```python
from build123d import *

# Parameters (mm, degrees)
SKETCH1_W                  = 40
SKETCH1_H                  = 22
BOSS_EXTRUDE1_DEPTH        = 11
SKETCH2_W                  = 40
SKETCH2_H                  = 22
SKETCH2_R                  = 7.843750423
BOSS_EXTRUDE2_DEPTH        = 5
SKETCH3_W                  = 24.5
SKETCH3_H                  = 15.5
CUT_EXTRUDE1_DEPTH         = 7.75
FILLET1_R                  = 7.75
SKETCH4_R                  = 5
CUT_EXTRUDE2_DEPTH         = 36.805900352
SKETCH5_W                  = 8
SKETCH5_H                  = 8
SKETCH5_R                  = 1.905800151
BOSS_EXTRUDE3_DEPTH        = 6
CUT_EXTRUDE3_START         = -3
SKETCH6_R                  = 3
SKETCH6_R_2                = 1.905800151
CUT_EXTRUDE3_DEPTH         = 3
SKETCH7_W                  = 16
SKETCH7_H                  = 16.5
BOSS_EXTRUDE5_DEPTH        = 28
MIRROR14_COPY_1_SKETCH_W   = 8
MIRROR14_COPY_1_SKETCH_H   = 8
MIRROR14_COPY_1_SKETCH_R   = 1.905800151
MIRROR14_COPY_1_DEPTH      = 6
MIRROR14_START             = -3
MIRROR14_COPY_2_SKETCH_R   = 3
MIRROR14_COPY_2_SKETCH_R_2 = 1.905800151
MIRROR14_COPY_2_DEPTH      = 3
FILLET1_OF_MIRROR14_R      = 7.75
SKETCH9_W                  = 28
SKETCH9_H                  = 3
BOSS_EXTRUDE6_DEPTH        = 18
CUT_EXTRUDE4_DEPTH         = 10
CUT_EXTRUDE5_DEPTH         = 73.919476136
CUT_EXTRUDE5_DEPTH_BACK    = 73.919476136
SKETCH11_R                 = 1.75
CUT_EXTRUDE6_DEPTH         = 76.121568141
CUT_EXTRUDE6_DEPTH_BACK    = 76.121568141
SKETCH12_R                 = 1.75
CUT_EXTRUDE9_DEPTH         = 12
CUT_EXTRUDE11_START        = -10
SKETCH16_R                 = 4
SKETCH16_R_2               = 1.75
SKETCH16_W                 = 10
SKETCH16_H                 = 6.5
CUT_EXTRUDE11_DEPTH        = 10
FILLET2_R                  = 2


# Some blends are built 0.0001 mm under size
with BuildPart() as part:
    # Sketch1 → Boss-Extrude1 (new body)
    with BuildSketch(Plane(origin=(0, 0, 0), x_dir=(1, 0, 0), z_dir=(0, 1, 0))):
        Rectangle(SKETCH1_W, SKETCH1_H)
    boss_extrude1 = extrude(amount=BOSS_EXTRUDE1_DEPTH)

    # Sketch2 → Boss-Extrude2 (add)
    with BuildSketch(Plane(origin=(0, 0, 0), x_dir=(1, 0, 0), z_dir=(0, 1, 0))):
        Rectangle(SKETCH2_W, SKETCH2_H)
        with Locations(Location((0, 0, 0), (0, 0, 270))):
            Circle(SKETCH2_R, mode=Mode.SUBTRACT)
    boss_extrude2 = extrude(amount=-BOSS_EXTRUDE2_DEPTH)

    # Sketch3 → Cut-Extrude1 (cut)
    with BuildSketch(Plane(origin=(0, 11, 0), x_dir=(1, 0, 0), z_dir=(0, 1, 0))):
        Rectangle(SKETCH3_W, SKETCH3_H)
    cut_extrude1 = extrude(amount=-CUT_EXTRUDE1_DEPTH, mode=Mode.SUBTRACT)

    # Fillet1
    fillet1_edges = [part.edges().sort_by_distance(p)[0] for p in [
        (0, 3.25, 7.75),
        (0, 3.25, -7.75),
    ]]
    fillet(fillet1_edges, radius=FILLET1_R - 0.0001)  # a hair under: the kernel refuses the full size

    # Sketch4 → Cut-Extrude2 (cut, symmetric)
    with BuildSketch(Plane(origin=(-12.25, 0, 0), x_dir=(0, 0, -1), z_dir=(1, 0, 0))):
        with Locations((0, 11)):
            Circle(SKETCH4_R)
    cut_extrude2 = extrude(amount=CUT_EXTRUDE2_DEPTH, both=True, mode=Mode.SUBTRACT)

    # Sketch5 → Boss-Extrude3 (add)
    with BuildSketch(Plane(origin=(0, 11, 0), x_dir=(1, 0, 0), z_dir=(0, 1, 0))):
        with Locations((16, -15)):
            Rectangle(SKETCH5_W, SKETCH5_H)
        with Locations(Location((16, -15, 0), (0, 0, 270))):
            Circle(SKETCH5_R, mode=Mode.SUBTRACT)
    boss_extrude3 = extrude(amount=-BOSS_EXTRUDE3_DEPTH)

    # Sketch6 → Cut-Extrude3 (cut)
    with BuildSketch(Plane.XZ.offset(-5).offset(CUT_EXTRUDE3_START)):
        with Locations(Location((16, 15, 0), (0, 0, 270))):
            Circle(SKETCH6_R)
        with Locations(Location((16, 15, 0), (0, 0, 90))):
            Circle(SKETCH6_R_2, mode=Mode.SUBTRACT)
    cut_extrude3 = extrude(amount=CUT_EXTRUDE3_DEPTH, mode=Mode.SUBTRACT)

    # Mirror8: Boss-Extrude3, Cut-Extrude3 across plane
    add(boss_extrude3.mirror(Plane(origin=(0, 0, 0), x_dir=(0, 0, 1), z_dir=(1, 0, 0))))
    add(cut_extrude3.mirror(Plane(origin=(0, 0, 0), x_dir=(0, 0, 1), z_dir=(1, 0, 0))), mode=Mode.SUBTRACT)

    # Sketch7 → Boss-Extrude5 (add)
    with BuildSketch(Plane(origin=(0, 0, -11), x_dir=(-1, 0, 0), z_dir=(0, 0, -1))):
        with Locations((-12, 9.25)):
            Rectangle(SKETCH7_W, SKETCH7_H)
    extrude(amount=BOSS_EXTRUDE5_DEPTH)

    # Mirror14: Boss-Extrude1, Boss-Extrude2, Cut-Extrude1, Cut-Extrude2, Boss-Extrude3, Cut-Extrude3 across plane
    add(boss_extrude1.mirror(Plane.XY.offset(-25)))
    add(boss_extrude2.mirror(Plane.XY.offset(-25)))
    add(cut_extrude1.mirror(Plane.XY.offset(-25)), mode=Mode.SUBTRACT)
    add(cut_extrude2.mirror(Plane.XY.offset(-25)), mode=Mode.SUBTRACT)
    add(boss_extrude3.mirror(Plane.XY.offset(-25)))
    add(cut_extrude3.mirror(Plane.XY.offset(-25)), mode=Mode.SUBTRACT)

    # Mirror14 copy 1 sketch → Mirror14 copy 1 (add)
    with BuildSketch(Plane(origin=(0, 11, -50), x_dir=(-1, 0, 0), z_dir=(0, 1, 0))):
        with Locations((16, -15)):
            Rectangle(MIRROR14_COPY_1_SKETCH_W, MIRROR14_COPY_1_SKETCH_H)
        with Locations(Location((16, -15, 0), (0, 0, 270))):
            Circle(MIRROR14_COPY_1_SKETCH_R, mode=Mode.SUBTRACT)
    extrude(amount=-MIRROR14_COPY_1_DEPTH)

    # Mirror14 copy 2 sketch → Mirror14 copy 2 (cut)
    with BuildSketch(Plane(origin=(0, 5, -50), x_dir=(-1, 0, 0), z_dir=(0, -1, 0)).offset(MIRROR14_START)):
        with Locations(Location((16, 15, 0), (0, 0, 270))):
            Circle(MIRROR14_COPY_2_SKETCH_R)
        with Locations(Location((16, 15, 0), (0, 0, 90))):
            Circle(MIRROR14_COPY_2_SKETCH_R_2, mode=Mode.SUBTRACT)
    extrude(amount=MIRROR14_COPY_2_DEPTH, mode=Mode.SUBTRACT)

    # Fillet1 of Mirror14
    fillet1_of_mirror14_edges = [part.edges().sort_by_distance(p)[0] for p in [
        (0, 3.25, -57.75),
        (0, 3.25, -42.25),
    ]]
    fillet(fillet1_of_mirror14_edges, radius=FILLET1_OF_MIRROR14_R - 0.0001)  # a hair under: the kernel refuses the full size

    # Sketch9 → Boss-Extrude6 (add)
    with BuildSketch(Plane.ZY.offset(-4)):
        with Locations((-25, 2.5)):
            Rectangle(SKETCH9_W, SKETCH9_H)
    extrude(amount=BOSS_EXTRUDE6_DEPTH)

    # Sketch10 → Cut-Extrude4 (cut)
    with BuildSketch(Plane(origin=(0, 17.5, 0), x_dir=(1, 0, 0), z_dir=(0, 1, 0))):
        with BuildLine():
            Line((9, 26.25), (9, 23.75))
            Line((9, 23.75), (11.727178029, 23.75))
            ThreePointArc((11.727178029, 23.75), (11.931001031, 24.360286817), (12, 25))
            ThreePointArc((12, 25), (11.931001031, 25.639713183), (11.727178029, 26.25))
            Line((11.727178029, 26.25), (9, 26.25))
        make_face()
        with BuildLine():
            Line((11.727178029, 23.75), (9, 23.75))
            Line((9, 23.75), (9, 26.25))
            Line((9, 26.25), (11.727178029, 26.25))
            ThreePointArc((11.727178029, 26.25), (6, 25), (11.727178029, 23.75))
        make_face()
        with BuildLine():
            ThreePointArc((12, 25), (11.931001031, 24.360286817), (11.727178029, 23.75))
            Line((11.727178029, 23.75), (20, 23.75))
            Line((20, 23.75), (20, 26.25))
            Line((20, 26.25), (11.727178029, 26.25))
            ThreePointArc((11.727178029, 26.25), (11.931001031, 25.639713183), (12, 25))
        make_face()
    extrude(amount=-CUT_EXTRUDE4_DEPTH, mode=Mode.SUBTRACT)

    # Sketch11 → Cut-Extrude5 (cut, two sides: drawn at the far end of the back side and taken through both)
    with BuildSketch(Plane(origin=(0, 7.5, 0), x_dir=(1, 0, 0), z_dir=(0, 1, 0)).offset(-CUT_EXTRUDE5_DEPTH_BACK)):
        with Locations(Location((9, 25, 0), (0, 0, 270))):
            Circle(SKETCH11_R)
    extrude(amount=CUT_EXTRUDE5_DEPTH + CUT_EXTRUDE5_DEPTH_BACK, mode=Mode.SUBTRACT)

    # Sketch12 → Cut-Extrude6 (cut, two sides: drawn at the far end of the back side and taken through both)
    with BuildSketch(Plane.ZY.offset(-4).offset(-CUT_EXTRUDE6_DEPTH_BACK)):
        with Locations((-33, 11)):
            Circle(SKETCH12_R)
    extrude(amount=CUT_EXTRUDE6_DEPTH + CUT_EXTRUDE6_DEPTH_BACK, mode=Mode.SUBTRACT)

    # Sketch15 → Cut-Extrude9 (cut)
    with BuildSketch(Plane(origin=(20, 0, 0), x_dir=(0, 0, -1), z_dir=(1, 0, 0))):
        Polygon((33, 14.175426481), (30.25, 12.58771324), (30.25, 9.41228676), (33, 7.824573519), (35.75, 9.41228676), (35.75, 12.58771324), align=None)
    extrude(amount=-CUT_EXTRUDE9_DEPTH, mode=Mode.SUBTRACT)

    # Sketch16 → Cut-Extrude11 (cut)
    # profile 1 of 2: a face of its own
    with BuildSketch(Plane(origin=(20, 0, 0), x_dir=(0, 0, -1), z_dir=(1, 0, 0)).offset(CUT_EXTRUDE11_START)):
        with Locations((33, 11)):
            Circle(SKETCH16_R)
        with Locations((33, 11)):
            Circle(SKETCH16_R_2, mode=Mode.SUBTRACT)
    # profile 2 of 2: a face of its own
    with BuildSketch(Plane(origin=(20, 0, 0), x_dir=(0, 0, -1), z_dir=(1, 0, 0)).offset(CUT_EXTRUDE11_START)):
        with Locations((34, 14.25)):
            Rectangle(SKETCH16_W, SKETCH16_H)
    extrude(amount=CUT_EXTRUDE11_DEPTH, mode=Mode.SUBTRACT)

    # Chamfer3
    # the kernel refuses this chamfer: 2.5 mm, written as the material it takes off along each edge
    with BuildSketch(Plane(origin=(4.790141486, 11, -37), x_dir=(0, -0.9712202897009368, 0.23818301550116588), z_dir=(1, 0, 0))) as chamfer3_piece_1_section:
        with BuildLine():
            Line((1.641163776, 0), (-0.550057664, 2.010038976))
            Line((-0.550057664, 2.010038976), (-0.598618679, 1.998129825))
            ThreePointArc((-0.598618679, 1.998129825), (-0.296653042, 0.999716345), (-0.048561014, -0.011909151))
            Line((-0.048561014, -0.011909151), (0.011909151, -0.048561014))
            ThreePointArc((0.011909151, -0.048561014), (0.818444442, 0.062835502), (1.633479525, -0.049405994))
            Line((1.633479525, -0.049405994), (1.641163776, 0))
        make_face()
    chamfer3_piece_1 = extrude(amount=20.419717028, mode=Mode.PRIVATE)
    chamfer3_piece_1 = split(chamfer3_piece_1, bisect_by=Plane(origin=(10, 11.063270064, -39.03704072), z_dir=(-1, 0, 0)), keep=Keep.TOP, mode=Mode.PRIVATE)
    chamfer3_piece_1 = split(chamfer3_piece_1, bisect_by=Plane(origin=(7.395070743, 11.063270064, -39), z_dir=(0, 0, -1)), keep=Keep.TOP, mode=Mode.PRIVATE)
    add(chamfer3_piece_1, mode=Mode.SUBTRACT)
    with BuildSketch(Plane(origin=(10, 11, -37), x_dir=(0, -0.9712202897009377, 0.23818301550116178), z_dir=(1, 0, 0))) as chamfer3_piece_2_section:
        with BuildLine():
            Line((1.641163776, 0), (-0.550057664, 2.010038976))
            Line((-0.550057664, 2.010038976), (-0.598618679, 1.998129825))
            ThreePointArc((-0.598618679, 1.998129825), (-0.296653042, 0.999716345), (-0.048561014, -0.011909151))
            Line((-0.048561014, -0.011909151), (0.011909151, -0.048561014))
            ThreePointArc((0.011909151, -0.048561014), (0.818444442, 0.062835502), (1.633479525, -0.049405994))
            Line((1.633479525, -0.049405994), (1.641163776, 0))
        make_face()
    chamfer3_piece_2 = extrude(amount=15.209858514, mode=Mode.PRIVATE)
    chamfer3_piece_2 = split(chamfer3_piece_2, bisect_by=Plane(origin=(17.604929257, 10.514615405, -39), z_dir=(0, 0, 1)), keep=Keep.TOP, mode=Mode.PRIVATE)
    add(chamfer3_piece_2, mode=Mode.SUBTRACT)
    with BuildSketch(Plane(origin=(10, 11, -37), x_dir=(0, -0.9712202897009377, 0.23818301550116178), z_dir=(1, 0, 0))) as chamfer3_piece_3_section:
        with BuildLine():
            Line((1.641163776, 0), (-0.550057664, 2.010038976))
            Line((-0.550057664, 2.010038976), (-0.598618679, 1.998129825))
            ThreePointArc((-0.598618679, 1.998129825), (-0.296653042, 0.999716345), (-0.048561014, -0.011909151))
            Line((-0.048561014, -0.011909151), (0.011909151, -0.048561014))
            ThreePointArc((0.011909151, -0.048561014), (0.818444442, 0.062835502), (1.633479525, -0.049405994))
            Line((1.633479525, -0.049405994), (1.641163776, 0))
        make_face()
    chamfer3_piece_3 = extrude(amount=15.209858514, mode=Mode.PRIVATE)
    chamfer3_piece_3 = split(chamfer3_piece_3, bisect_by=Plane(origin=(17.604929257, 11.063270064, -39), z_dir=(0, 0, -1)), keep=Keep.TOP, mode=Mode.PRIVATE)
    add(chamfer3_piece_3, mode=Mode.SUBTRACT)

    # Fillet2
    fillet2_edges = [part.edges().sort_by_distance(p)[0] for p in [
        (11.727178029, 12.5, -23.75),
        (11.727178029, 12.5, -26.25),
    ]]
    fillet(fillet2_edges, radius=FILLET2_R)


solid = part.part
```
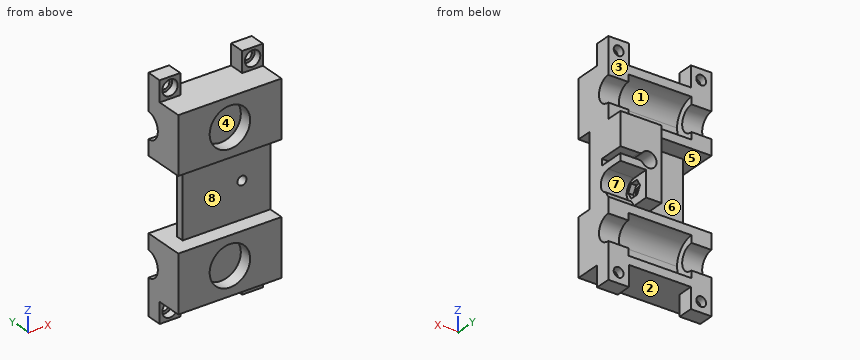
Build history of the part. All positions in model axes, mm. Face numbers are marked on the shaded views. A direction names the side the tool comes from. Round coordinates to 2 decimals unless told otherwise and drop trailing zeros. Loops run counter-clockwise (first coordinate to the right, second up) from the corner with the lowest first, then second, coordinate; pieces in that order, holes last.
Item 1: Two-plate mould, pull along Z, no slides. Class the marked faces 1, 2 and 3: released by +Z, released by -Z, zero draft, split by the parting line, or undercut.
Item 2: Saw through at A-A (z = -65). List the corners of the cut face in (x, y), then the cut area to 3 significant figures.
Item 3: Which spindle directions (+Z, -Z, +X, -X, +Y, -Y) get a long thin tool onto all of the face, cutting with end or side? Do the marked faces 4, 5, 6, 7 and 8. Say none if no direction does.
Item 4: Pin check, flat tips, straight feed: P1, Ø4.5, axis at y = 11, z = -33, coming from the +X side; P2, Ø1.8, axis at x = 7.5, z = -8, coming from the +Y side; P3, Ø13, axis at x = -0.5, y = 6.5, coming from the +Z side; P4, Ø3.5, axis at x = 16, z = -65, coming from the -Y side. Stop position of each tip, or through.
Item 5: Drill centre lines: line 1 along X through (y, z) = (7.3, 15); line 2 along X through (y, z) = (9.95, 15); line 3 along Y through (x, z) = (5, -33). Where is each one in solid material? Low to high.
Item 6: Saw through at C-C (y = 16.25). List the corners of the cut face in (x, z).
Worked answers:
1. face 1: undercut
1. face 2: released by -Z
1. face 3: zero draft
2. outline: (-20, 5) - (-19, 5) - (-19, 8) - (-17.91, 8) - (-17.91, 11) - (-20, 11) - close; (-14.09, 8) - (-13, 8) - (-13, 5) - (-12, 5) - (-12, 11) - (-14.09, 11) - close; (12, 5) - (13, 5) - (13, 8) - (14.09, 8) - (14.09, 11) - (12, 11) - close; (17.91, 8) - (19, 8) - (19, 5) - (20, 5) - (20, 11) - (17.91, 11) - close
2. area: 37.1 mm2
3. face 4: -Y
3. face 5: -X
3. face 6: -X, +Y
3. face 7: +X, +Y
3. face 8: +X, -X, -Y
4. P1: stops at x = 8
4. P2: stops at y = 11
4. P3: stops at z = 11
4. P4: passes through
5. line 1: x = -20 to -19, -13 to -12, 12 to 13, 19 to 20
5. line 2: x = -20 to -17.91, -14.09 to -12, 12 to 14.09, 17.91 to 20
5. line 3: y = 1 to 9.25, 12.75 to 17.5
6. outline: (4, -39) - (10, -39) - (10, -29) - (20, -29) - (20, -26.25) - (12.8, -26.25) arc R2 ccw to (11.28, -26.95) arc R3 cw (long way) to (11.28, -23.05) arc R2 ccw to (12.8, -23.75) - (20, -23.75) - (20, -11) - (4, -11) - close
